```python
from build123d import *

# Parameters (mm, degrees)
F1_DEPTH  = 22.225
F3_R      = 19.05
F4_DEPTH  = 20.32
F2_R      = 6.35
F6_DEPTH  = 38.1
F5_W      = 17.78
F5_H      = 38.1
F7_DEPTH  = 19.05
F8_SIZE   = 2.54
F10_DEPTH = 7.62
F11_R     = 6.35
F12_DEPTH = 26.67
F13_SIZE  = 1.27
F15_DEPTH = 38.1
F16_W     = 5.08
F16_H     = 40.64
F17_DEPTH = 25.4
F18_R     = 6.35
F19_DEPTH = 19.05
F20_R     = 1.905
F20_R_2   = 1.27
F20_R_3   = 2.54
F20_R_4   = 3.175
F21_DEPTH = 12.7
F22_SIZE  = 1.27


with BuildPart() as f1:
    # F0 (on Front) → F1 (new body, symmetric)
    with BuildSketch(Plane.XZ):
        with BuildLine():
            Line((7.62, 0), (-7.62, 0))
            Line((-7.62, 0), (-7.62, -24.5142909701))
            Line((-7.62, -24.5142909701), (-7.62, -27.8114224211))
            ThreePointArc((-7.62, -27.8114224211), (-8.3544623748, -30.77591853), (-10.3879487179, -33.0546474413))
            ThreePointArc((-10.3879487179, -33.0546474413), (-16.2850591132, -39.6629612843), (-18.415, -48.26))
            Line((-18.415, -48.26), (-18.415, -64.516))
            ThreePointArc((-18.415, -64.516), (-17.9686307345, -65.5936307345), (-16.891, -66.04))
            Line((-16.891, -66.04), (-16.764, -66.04))
            ThreePointArc((-16.764, -66.04), (-15.6863692655, -65.5936307345), (-15.24, -64.516))
            Line((-15.24, -64.516), (-15.24, -48.26))
            ThreePointArc((-15.24, -48.26), (0, -33.02), (15.24, -48.26))
            Line((15.24, -48.26), (15.24, -65.0540764831))
            ThreePointArc((15.24, -65.0540764831), (15.6863692655, -66.1317072176), (16.764, -66.5780764831))
            Line((16.764, -66.5780764831), (16.891, -66.5780764831))
            ThreePointArc((16.891, -66.5780764831), (17.9686307345, -66.1317072176), (18.415, -65.0540764831))
            Line((18.415, -65.0540764831), (18.415, -48.26))
            ThreePointArc((18.415, -48.26), (16.2850591132, -39.6629612843), (10.3879487179, -33.0546474413))
            ThreePointArc((10.3879487179, -33.0546474413), (8.3544623748, -30.77591853), (7.62, -27.8114224211))
            Line((7.62, -27.8114224211), (7.62, -24.5142909701))
            Line((7.62, -24.5142909701), (7.62, 0))
        make_face()
    extrude(amount=F1_DEPTH, both=True)

    # F3 (on Right) → F4 (join, symmetric)
    with BuildSketch(Plane.YZ):
        with Locations((0, -66.04)):
            Circle(F3_R)
    extrude(amount=F4_DEPTH, both=True)

    # F2 (on Right) → F6 (cut, symmetric)
    with BuildSketch(Plane.YZ):
        with Locations((0, -66.04)):
            Circle(F2_R)
    extrude(amount=F6_DEPTH, both=True, mode=Mode.SUBTRACT)

    # F5 (on Front) → F7 (cut, symmetric)
    with BuildSketch(Plane.XZ):
        with Locations((0, -66.04)):
            Rectangle(F5_W, F5_H)
    extrude(amount=F7_DEPTH, both=True, mode=Mode.SUBTRACT)

    # F8
    f8_edges = [f1.edges().sort_by_distance(p)[0] for p in [
        (-8.89, -19.05, -66.04),
        (8.89, -19.05, -66.04),
    ]]
    chamfer(f8_edges, length=F8_SIZE)

    # F9 (on Right) → F10 (join, symmetric)
    with BuildSketch(Plane.YZ):
        with BuildLine():
            Line((19.0499954742, -0.0131314098), (19.0499954742, 38.0868685902))
            ThreePointArc((19.0499954742, 38.0868685902), (0, 57.15), (-19.0499954742, 38.0868685902))
            Line((-19.0499954742, 38.0868685902), (-19.0499954742, -0.0131314098))
            Line((-19.0499954742, -0.0131314098), (19.0499954742, -0.0131314098))
        make_face()
    extrude(amount=F10_DEPTH, both=True)

    # F11 (on Right) → F12 (join)
    with BuildSketch(Plane.YZ):
        with Locations((0, 38.1)):
            Circle(F11_R)
    extrude(amount=F12_DEPTH)

    # F13
    f13_edges = [f1.edges().sort_by_distance(p)[0] for p in [
        (26.67, -6.35, 38.1),
    ]]
    chamfer(f13_edges, length=F13_SIZE)

    # F14 (on Right) → F15 (intersect, symmetric)
    with BuildSketch(Plane.YZ):
        with BuildLine():
            ThreePointArc((17.184531987, -57.8184210526), (7.235369251, -13.97), (17.184531987, 29.8784210526))
            ThreePointArc((17.184531987, 29.8784210526), (0, 57.15), (-17.184531987, 29.8784210526))
            ThreePointArc((-17.184531987, 29.8784210526), (-7.235369251, -13.97), (-17.184531987, -57.8184210526))
            ThreePointArc((-17.184531987, -57.8184210526), (0, -85.09), (17.184531987, -57.8184210526))
        make_face()
    extrude(amount=F15_DEPTH, both=True, mode=Mode.INTERSECT)

    # F16 (on Front) → F17 (cut, symmetric)
    with BuildSketch(Plane.XZ):
        Rectangle(F16_W, F16_H)
    extrude(amount=F17_DEPTH, both=True, mode=Mode.SUBTRACT)

    # F18 (on face) → F19 (join)
    with BuildSketch(Plane(origin=(-7.62, 0, 0), x_dir=(0, -1, 0), z_dir=(-1, 0, 0))):
        with Locations((0, 38.1)):
            Circle(F18_R)
    extrude(amount=F19_DEPTH)

    # F20 (on Right) → F21 (cut, symmetric)
    with BuildSketch(Plane.YZ):
        with Locations((0, -3.81)):
            Circle(F20_R)
        with Locations((0, -9.525)):
            Circle(F20_R_2)
        with Locations((0, -14.605)):
            Circle(F20_R_2)
        with Locations((0, 3.175)):
            Circle(F20_R_3)
        with Locations((0, 11.43)):
            Circle(F20_R_4)
    extrude(amount=F21_DEPTH, both=True, mode=Mode.SUBTRACT)

    # F22
    f22_edges = [f1.edges().sort_by_distance(p)[0] for p in [
        (-26.67, 6.35, 38.1),
    ]]
    chamfer(f22_edges, length=F22_SIZE)


with BuildPart() as f1_1:
    # F24: moved
    add(f1.part.moved(Location((0, 0, -38.1))))


solid = f1_1.part
```
The model under review builds one solid part; all positions refer to its coordinate system, in mm. A direction names the side the tool comes from. Round coordinates to 2 decimals unless told otherwise and drop trailing zeros. Loops run counter-clockwise (first coordinate to the right, second up) from the corner with the lowest first, then second, coordinate; pieces in that order, holes last. Notation, with made-up numbers: (56, -4) -> (60, -4) arc R15 ccw to (60, 1) -> close; hole circle Ø9 at (-22, 32.5). An arc over 180 degrees is marked (long way). Answer as a JSON object with one key per item and string values. Group by question number.
1) We need section B-B on y = 0. Give the number of separate pieces and of enclosed holes in the cut face, then the cut area to 3 significant figures.
2) For pin 1 Ø6 at (y, z) = (0, -34.925) entering from +X; pin 2 Ø1.5 at (y, z) = (8, -84.5) entering from +X; pin 3 Ø6 at (x, y) = (11, -14.5) entering from -Z; pin 4 Ø8 at (x, z) = (-15.5, -51) entering from +Y, all flat-tipped, find the tip position at first contact; note any pin that passes through.
3) We need section D-D on z = -41.91. Write out the cut boundary in (x, y) (3 decimals).
4) For line 1 (X direction, y = 10.5, z = -112); line 2 (X direction, y = 11, z = -19); line 3 (Z direction, x = -6, y = 0) (3 decimals), list the stretches that pass through material, from the lowest coordinate up. Write a range as [from, to].
5) For faces 1 (the face through (7.62, 0, -15)), 2 (the face through (-15.24, -12, -89)), 3 (the face through (-16.4, 0.8, 6.3)), 4 (the face through (-20.32, 0, -112)), 5 (the face through (8.375, -0.127, -68.914)), list the 3-axis set-ups (+Z, -Z, +X, -X, +Y, -Y) from which the entire face can be reached by the end or side of a thin tool; tool diameter is ignored.
6) We need section A-A on z = -26.67. Write out the cut boundary in (x, y) (3 decimals).
7) Mouldability with a two-part tool opening along X and no side actions: class faces 6 (the face through (-0.335, -0.185, -71.124)), 7 (the face through (20.32, 0, -112)), 8 (the face through (5.04, -0.41, -43.77)), 9 (the face through (-8.334, -0.127, -68.838)) as released by +X, released by -X, zero draft, split by the parting line, or undercut.
Result set:
{
 "1": {"separate pieces": "12", "enclosed holes": "0", "area": "2,130 mm²"},
 "2": {"pin 1": "x = 7.62", "pin 2": "x = 18.38", "pin 3": "z = -119.3", "pin 4": "through"},
 "3": {"outline": "(-7.62, -7.745) -> (-2.54, -7.745) -> (-2.54, -1.905) -> (-7.62, -1.905) -> close; (-7.62, 1.905) -> (-2.54, 1.905) -> (-2.54, 7.745) -> (-7.62, 7.745) -> close; (2.54, -7.745) -> (7.62, -7.745) -> (7.62, -1.905) -> (2.54, -1.905) -> close; (2.54, 1.905) -> (7.62, 1.905) -> (7.62, 7.745) -> (2.54, 7.745) -> close"},
 "4": {"line 1": "[-20.32, -8.89], [8.89, 20.32]", "line 2": "[-7.62, -2.54], [2.54, 7.62]", "line 3": "[-72.351, -53.975], [-51.435, -48.895], [-46.355, -43.815], [-40.005, -37.465], [-32.385, -29.845], [-23.495, 19.05]"},
 "5": {"face 1": "+X", "face 2": "-Y", "face 3": "-X", "face 4": "-Z, -X, +Y, -Y", "face 5": "+X, +Y, -Y"},
 "6": {"outline": "(-7.62, -10.462) -> (-2.54, -10.462) -> (-2.54, -3.175) -> (-7.62, -3.175) -> close; (-7.62, 3.175) -> (-2.54, 3.175) -> (-2.54, 10.462) -> (-7.62, 10.462) -> close; (2.54, -10.462) -> (7.62, -10.462) -> (7.62, -3.175) -> (2.54, -3.175) -> close; (2.54, 3.175) -> (7.62, 3.175) -> (7.62, 10.462) -> (2.54, 10.462) -> close"},
 "7": {"face 6": "undercut", "face 7": "released by +X", "face 8": "zero draft", "face 9": "released by -X"}
}
